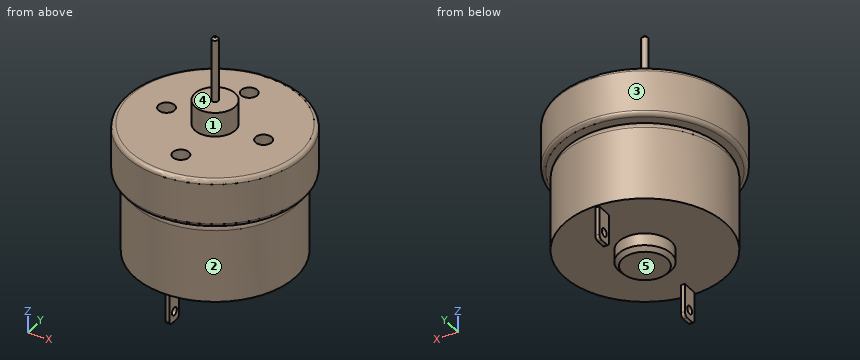
```python
from build123d import *

# Parameters (mm, degrees)
SKETCH1_R            = 10
BOSS_EXTRUDE1_DEPTH  = 10
FILLET1_R            = 1
SKETCH2_R            = 3.25
BOSS_EXTRUDE2_DEPTH  = 2
SKETCH3_W            = 0.5
SKETCH3_H            = 2
BOSS_EXTRUDE4_DEPTH  = 4
SKETCH5_R            = 0.5
CUT_EXTRUDE2_DEPTH   = 4
FILLET3_R            = 0.5
FILLET3_OF_MIRROR2_R = 0.5
SKETCH6_R            = 11
BOSS_EXTRUDE5_DEPTH  = 6
FILLET4_R            = 0.5
SKETCH7_R            = 2.5
BOSS_EXTRUDE6_DEPTH  = 3
SKETCH8_R            = 0.4
BOSS_EXTRUDE7_DEPTH  = 8
CHAMFER1_SIZE        = 0.5
CHAMFER2_SIZE        = 0.25
SKETCH16_R           = 1
CUT_EXTRUDE3_DEPTH   = 8


with BuildPart() as part:
    # Sketch1 → Boss-Extrude1 (new body)
    with BuildSketch(Plane.XY):
        Circle(SKETCH1_R)
    extrude(amount=BOSS_EXTRUDE1_DEPTH)

    # Fillet1
    fillet1_edges = [part.edges().sort_by_distance(p)[0] for p in [
        (-10, 0, 10),
    ]]
    fillet(fillet1_edges, radius=FILLET1_R)

    # Sketch2 → Boss-Extrude2 (add)
    with BuildSketch(Plane(origin=(0, 0, 0), x_dir=(-1, 0, 0), z_dir=(0, 0, -1))):
        Circle(SKETCH2_R)
    extrude(amount=BOSS_EXTRUDE2_DEPTH)

    # Sketch3 → Boss-Extrude4 (add)
    with BuildSketch(Plane(origin=(0, 0, 0), x_dir=(-1, 0, 0), z_dir=(0, 0, -1))):
        with Locations((0, 8.75)):
            Rectangle(SKETCH3_W, SKETCH3_H)
    boss_extrude4 = extrude(amount=BOSS_EXTRUDE4_DEPTH)

    # Sketch5 → Cut-Extrude2 (cut)
    with BuildSketch(Plane.ZY.offset(0.25)):
        with Locations(Location((-2.75, 8.75, 0), (0, 0, 270))):
            Circle(SKETCH5_R)
    cut_extrude2 = extrude(amount=-CUT_EXTRUDE2_DEPTH, mode=Mode.SUBTRACT)

    # Fillet3
    fillet3_edges = [part.edges().sort_by_distance(p)[0] for p in [
        (0, 9.75, -4),
        (0, 7.75, -4),
    ]]
    fillet(fillet3_edges, radius=FILLET3_R)

    # Mirror2: Boss-Extrude4, Cut-Extrude2 across plane
    add(boss_extrude4.mirror(Plane.ZX))
    add(cut_extrude2.mirror(Plane.ZX), mode=Mode.SUBTRACT)

    # Fillet3 of Mirror2
    fillet3_of_mirror2_edges = [part.edges().sort_by_distance(p)[0] for p in [
        (0, -9.75, -4),
        (0, -7.75, -4),
    ]]
    fillet(fillet3_of_mirror2_edges, radius=FILLET3_OF_MIRROR2_R)

    # Sketch6 → Boss-Extrude5 (add)
    with BuildSketch(Plane.XY.offset(10)):
        Circle(SKETCH6_R)
    extrude(amount=BOSS_EXTRUDE5_DEPTH)

    # Fillet4
    fillet4_edges = [part.edges().sort_by_distance(p)[0] for p in [
        (-11, 0, 10),
        (-11, 0, 16),
    ]]
    fillet(fillet4_edges, radius=FILLET4_R)

    # Sketch7 → Boss-Extrude6 (add)
    with BuildSketch(Plane.XY.offset(16)):
        Circle(SKETCH7_R)
    extrude(amount=BOSS_EXTRUDE6_DEPTH)

    # Sketch8 → Boss-Extrude7 (add)
    with BuildSketch(Plane.XY.offset(19)):
        Circle(SKETCH8_R)
    extrude(amount=BOSS_EXTRUDE7_DEPTH)

    # Chamfer1
    chamfer1_edges = [part.edges().sort_by_distance(p)[0] for p in [
        (3.25, 0, -2),
    ]]
    chamfer(chamfer1_edges, length=CHAMFER1_SIZE)

    # Chamfer2
    chamfer2_edges = [part.edges().sort_by_distance(p)[0] for p in [
        (-0.4, 0, 27),
    ]]
    chamfer(chamfer2_edges, length=CHAMFER2_SIZE)

    # Sketch16 → Cut-Extrude3 (cut)
    with BuildSketch(Plane.XY.offset(16)):
        with Locations((0, 7)):
            Circle(SKETCH16_R)
        with Locations((0, -7)):
            Circle(SKETCH16_R)
        with Locations((6, 0)):
            Circle(SKETCH16_R)
        with Locations(Location((-6, 0, 0), (0, 0, 180))):
            Circle(SKETCH16_R)
    extrude(amount=-CUT_EXTRUDE3_DEPTH, mode=Mode.SUBTRACT)


solid = part.part
```
Input: part model. Units: mm. Frame: model coordinates. Face numbers are marked on the shaded views. A direction names the side the tool comes from. Give positions to 0.01 mm unless a question says otherwise; leave off trailing zeros. Loops run counter-clockwise (first coordinate to the right, second up) from the corner with the lowest first, then second, coordinate; pieces in that order, holes last.
1) Section query B-B on z = 6.5. Return the cut outline in (x, y), and give its area (3 significant figures).
A:
outline: circle Ø20 at (0, 0)
area: 314 mm2
2) Contact query for flat-ended pins moving along their axis: pin 1 (12 mm diameter, centred on y = 0, z = 3.5, fed in from -X); pin 2 (10 mm diameter, centred on x = -7, z = 16, fed in from +Y); pin 3 (0.6 mm diameter, centred on x = 6, y = 0, fed in from +Z). Output: stop coordinate, or through.
A:
pin 1: stops at x = -10
pin 2: stops at y = 10.81
pin 3: stops at z = 8
3) Line query: L1, parallel to Z at x = 0, y = 8.75; L2, parallel to Z at x = 4, y = -2.75; L3, parallel to Y at x = -6, z = 14. Output: solid intervals per line, ascending.
A:
L1: z = -4 to -3.25, -2.25 to 16
L2: z = 0 to 16
L3: y = -9.22 to -1, 1 to 9.22
4) Section query A-A on z = -2.75. Return the cut outline in (x, y), and give its area (3 significant figures).
A:
outline: (-0.25, -9.75) - (0.25, -9.75) - (0.25, -9.25) - (-0.25, -9.25) - close; (-0.25, -8.25) - (0.25, -8.25) - (0.25, -7.75) - (-0.25, -7.75) - close; (-0.25, 7.75) - (0.25, 7.75) - (0.25, 8.25) - (-0.25, 8.25) - close; (-0.25, 9.25) - (0.25, 9.25) - (0.25, 9.75) - (-0.25, 9.75) - close
area: 1.00 mm2
5) Mould query, pull axis Y, two halves, no side actions, for the marked faces 3, 4 and 5. Classes: released by +Y, released by -Y, zero draft, split by the parting line, or undercut.
A:
face 3: split by the parting line
face 4: zero draft
face 5: undercut
6) Section query C-C on z = 19.5. Return the cut outline in (x, y), and give its area (3 significant figures).
A:
outline: circle Ø0.8 at (0, 0)
area: 0.503 mm2
7) Reachability of the marked faces 1 and 2 from +Z, -Z, +X, -X, +Y, -Y: full face, straight path, thin tool, end or side. Return the list, or none.
A:
face 1: +Z
face 2: -Z
